Work out the finished part from the listing and answer in its coordinate system (mm). A direction names the side the tool comes from. Give positions to 0.01 mm unless a question says otherwise; leave off trailing zeros. Order: outer loops, then holes, each group sorted by start corner. A loop starts at its lowest first (then second) coordinate and runs counter-clockwise, first axis right, second up.
```python
from build123d import *

# Parameters (mm, degrees)
SKETCH1_R           = 6.35
BOSS_EXTRUDE1_DEPTH = 12.7


with BuildPart() as part:
    # Sketch1 → Boss-Extrude1 (new body)
    with BuildSketch(Plane(origin=(0, 0, 0), x_dir=(1, 0, 0), z_dir=(0, 1, 0))):
        with BuildLine():
            Line((171.45, 10.16), (26.09574153, 126.443406776))
            ThreePointArc((26.09574153, 126.443406776), (25.34977374, 126.856815931), (24.509016109, 127))
            Line((24.509016109, 127), (2.54, 127))
            ThreePointArc((2.54, 127), (0.743948776, 126.256051224), (0, 124.46))
            Line((0, 124.46), (0, 72.055027479))
            Line((0, 72.055027479), (-63.5, 9.332908944))
            Line((-63.5, 9.332908944), (-101.6, 9.332908944))
            Line((-101.6, 9.332908944), (-101.6, -0.827091056))
            Line((-101.6, -0.827091056), (203.2, 0))
            Line((203.2, 0), (203.2, 10.16))
            Line((203.2, 10.16), (171.45, 10.16))
        make_face()
        with Locations(Location((12.7, 88.9, 0), (0, 0, 90))):
            Circle(SKETCH1_R, mode=Mode.SUBTRACT)
        with Locations(Location((12.7, 44.45, 0), (0, 0, 90))):
            Circle(SKETCH1_R, mode=Mode.SUBTRACT)
        Polygon((0, 9.525), (0, 58.085027479), (-48.962001116, 9.525), align=None, mode=Mode.SUBTRACT)
        Polygon((25.4, 9.525), (25.4, 110.49), (139.7, 19.05), (139.7, 9.525), align=None, mode=Mode.SUBTRACT)
    extrude(amount=BOSS_EXTRUDE1_DEPTH)


solid = part.part
```
1. Which of the six approach directions +Z, -Z, +X, -X, +Y, -Y give full straight-line access (tool end or side, diameter ignored) to faces 1 (the face through (-24.138, 6.261, -34.145)), 2 (the face through (99.79, 6.26, -67.49)), 3 (the face through (-82, 6, -9.333))?
Findings below:
face 1: +Y, -Y
face 2: -Z, +X, +Y, -Y
face 3: -Z, -X, +Y, -Y
2. The part is cut by section C-C (y = 4.25). Write down the section's boundary in (x, z) (3 decimals).
Findings below:
outline: (-101.6, -9.333) - (-63.5, -9.333) - (0, -72.055) - (0, -124.46) arc R2.54 ccw to (2.54, -127) - (24.509, -127) arc R2.54 ccw to (26.096, -126.443) - (171.45, -10.16) - (203.2, -10.16) - (203.2, 0) - (-101.6, 0.827) - close; hole (-48.962, -9.525) - (0, -58.085) - (0, -9.525) - close; hole circle Ø12.7 at (12.7, -88.9); hole circle Ø12.7 at (12.7, -44.45); hole (25.4, -110.49) - (139.7, -19.05) - (139.7, -9.525) - (25.4, -9.525) - close
3. The mould has two halves that part along Z. Classify faces 4 (the face through (25.4, 6, -59)), 5 (the face through (-101.6, 6, -4)), 6 (the face through (139.7, 6, -14)), 7 (the face through (188, 6, -10.16)): pulls with the +Z half, pulls with the -Z half, needs draft (parallel to the pull), parting line crosses it, or undercut.
Findings below:
face 4: undercut
face 5: needs draft
face 6: undercut
face 7: pulls with the -Z half
4. The part is cut by section B-B (z = -47). Write down the section's boundary in (x, y), then the cut area to 3 significant figures.
Findings below:
outline: (-25.37, 0) - (-11.18, 0) - (-11.18, 12.7) - (-25.37, 12.7) - close; (0, 0) - (6.88, 0) - (6.88, 12.7) - (0, 12.7) - close; (18.52, 0) - (25.4, 0) - (25.4, 12.7) - (18.52, 12.7) - close; (104.76, 0) - (125.4, 0) - (125.4, 12.7) - (104.76, 12.7) - close
area: 617 mm2
5. The part is cut by section D-D (z = -28). Write down the section's boundary in (x, y).
Findings below:
outline: (-44.6, 0) - (-30.33, 0) - (-30.33, 12.7) - (-44.6, 12.7) - close; (0, 0) - (25.4, 0) - (25.4, 12.7) - (0, 12.7) - close; (128.51, 0) - (149.15, 0) - (149.15, 12.7) - (128.51, 12.7) - close
6. Given P1, Ø6.5, axis at y = 9, z = -55.5, coming from the +X side; P2, Ø4, axis at x = -18.5, y = 6.5, coming from the -Z side; P3, Ø4, axis at x = 87.5, y = 4.5, coming from the -Z side; P4, Ø16.5, axis at x = 12.7, z = -88.9, coming from the +Y side, each flat-ended and moving along its own axis, determine where each tip first touches the part or whether it passes through.
Findings below:
P1: stops at x = 118.84
P2: stops at z = -55.76
P3: stops at z = -78.92
P4: stops at y = 12.7
7. The part is cut by section A-A (x = 80.5). Write down the section's boundary in (y, z) (3 decimals).
Findings below:
outline: (0, -82.92) - (12.7, -82.92) - (12.7, -66.41) - (0, -66.41) - close; (0, -9.525) - (12.7, -9.525) - (12.7, 0.333) - (0, 0.333) - close
8. Straight lines are drawn through the part: probe 1 along X at (y, z) = (4.5, -87.5) (1 decimal); probe 2 along X at (y, z) = (2.75, -10); probe 3 along X at (y, z) = (8.75, -44.45). For each, find the intervals that lie inside material, in ascending order.
Findings below:
probe 1: x = 0 to 6.5, 18.9 to 25.4, 54.1 to 74.8
probe 2: x = -62.82 to -48.48, 0 to 25.4, 139.7 to 203.2
probe 3: x = -27.95 to -13.75, 0 to 6.35, 19.05 to 25.4, 107.95 to 128.59
